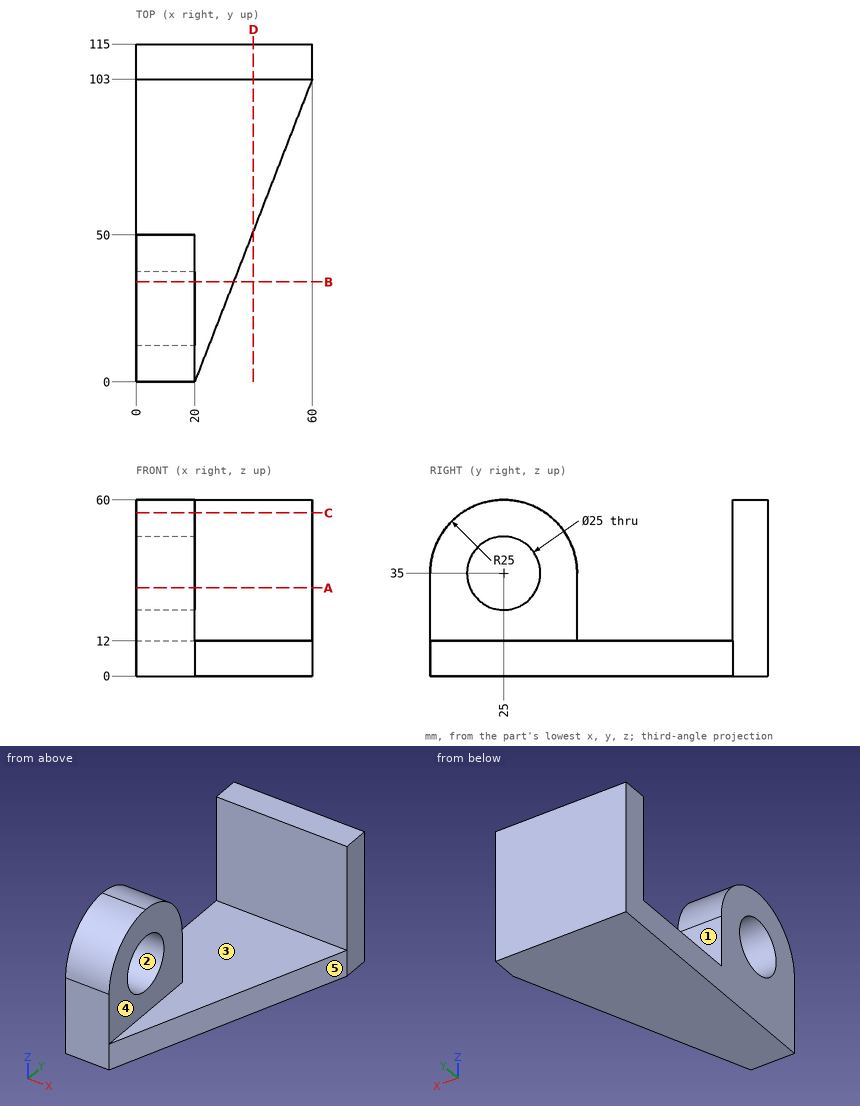
Geometry check sheet. Reference: drawing and pictorial views, mm from the part's lowest x, y, z. A direction names the side the tool comes from. Give positions to 0.01 mm unless a question says otherwise; leave off trailing zeros. Write each loop counter-clockwise with the first axis right and the second up, starting at its lowest first coordinate (ties: lowest second). Pieces come first, ordered by that corner, then holes. Notation, with made-up numbers: M 80,81 L 122,81 A15 ccw 122,86 Z; hole C 5,-2 d1. An arc over 180 degrees is marked long. Use CSV: the item, a comma, the result in double quotes.
1) Cross-section at C-C (z = 55.5). Enter the section's corners in (x, y), plus the area to 3 significant figures.
Final values:
outline,"M 0,10.69 L 20,10.69 L 20,39.31 L 0,39.31 Z; M 0,103 L 60,103 L 60,115 L 0,115 Z"
area,"1,290 mm²"
2) Cross-section at D-D (x = 40). Enter the section's corners in (y, z).
Final values:
outline,"M 51.5,0 L 115,0 L 115,60 L 103,60 L 103,12 L 51.5,12 Z"
3) Cross-section at B-B (y = 34). Enter the section's corners in (x, z).
Final values:
outline,"M 0,0 L 33.2,0 L 33.2,12 L 20,12 L 20,26.33 L 0,26.33 Z; M 0,43.67 L 20,43.67 L 20,58.32 L 0,58.32 Z"
4) Access from +Z, -Z, +X, -X, +Y, -Y to the whole of each face (thin tool, end or side, straight path). Record for the marked faces 1 and 2.
Final values:
face 1,"+Z, +X, -X"
face 2,"+X, -X"
5) Cross-section at A-A (z = 30). Enter the section's corners in (x, y), plus the area to 3 significant figures.
Final values:
outline,"M 0,0 L 20,0 L 20,13.54 L 0,13.54 Z; M 0,36.46 L 20,36.46 L 20,50 L 0,50 Z; M 0,103 L 60,103 L 60,115 L 0,115 Z"
area,"1,260 mm²"
6) Go/stop test with flat-tipped pins: pin 1 Ø4 at (x, y) = (6, 28.5) entering from +Z; pin 2 Ø2 at (y, z) = (100, 8.5) entering from +X; pin 3 Ø1 at (x, y) = (41, 83) entering from +Z. Record where each tip stops, or that it passes through.
Final values:
pin 1,"z = 59.95"
pin 2,"x = 59.22"
pin 3,"z = 12"
7) Release check for a two-part mould opening along Y. For the marked faces 3, 4 and 5 record: released by +Y, released by -Y, zero draft, split by the parting line, or undercut.
Final values:
face 3,"undercut"
face 4,"zero draft"
face 5,"released by -Y"
8) Material ranges on line 1 along Z through (x, y) = (36, 88); line 2 along Y through (x, z) = (40.5, 38.5); line 3 along X through (y, z) = (7, 23), recorded low to high.
Final values:
line 1,"0 to 12"
line 2,"103 to 115"
line 3,"0 to 20"
